from build123d import *

# Parameters (mm, degrees)
F1_DEPTH = 60
F2_SIZE  = 40
F3_R     = 90
F4_DEPTH = 10
F5_W     = 43
F5_H     = 43
F6_DEPTH = 40
F7_R     = 4
F8_DEPTH = 10


with BuildPart() as f1:
    # F0 (on Top) → F1 (new body)
    with BuildSketch(Plane.XY):
        Polygon((-173.205081, -100), (173.205081, -100), (0, 200), align=None)
    extrude(amount=F1_DEPTH)

    # F2
    f2_edges = [f1.edges().sort_by_distance(p)[0] for p in [
        (-173.205081, -100, 30),
        (173.205081, -100, 30),
        (0, 200, 30),
    ]]
    chamfer(f2_edges, length=F2_SIZE)

    # F3 (on face) → F4 (join)
    with BuildSketch(Plane.XY.offset(60)):
        Circle(F3_R)
    extrude(amount=F4_DEPTH)

    # F5 (on face) → F6 (cut)
    with BuildSketch(Plane.XY.offset(60)):
        with Locations((0, 130.358984)):
            Rectangle(F5_W, F5_H)
        Polygon((-120.763738, -94.549038), (-83.524645, -73.049038), (-105.024645, -35.809946), (-142.263738, -57.309946), align=None)
        Polygon((142.263738, -57.309946), (105.024645, -35.809946), (83.524645, -73.049038), (120.763738, -94.549038), align=None)
    extrude(amount=-F6_DEPTH, mode=Mode.SUBTRACT)

    # F7 (on face) → F8 (cut)
    with BuildSketch(Plane.XY.offset(60)):
        with Locations((-29.5, 130.358984)):
            Circle(F7_R)
        with Locations((29.5, 130.358984)):
            Circle(F7_R)
        with Locations((-98.144192, -90.727241)):
            Circle(F7_R)
        with Locations((-127.644192, -39.631743)):
            Circle(F7_R)
        with Locations((127.644192, -39.631743)):
            Circle(F7_R)
        with Locations((98.144192, -90.727241)):
            Circle(F7_R)
    extrude(amount=-F8_DEPTH, mode=Mode.SUBTRACT)


solid = f1.part
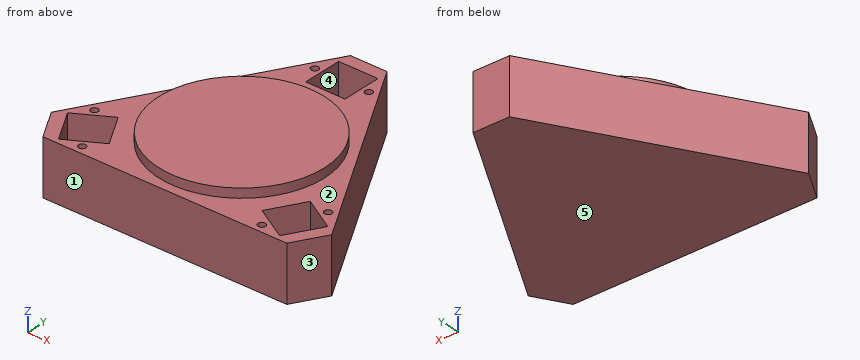
Verification items for the finished model (mm, model axes). Face numbers are marked on the shaded views. A direction names the side the tool comes from. Coordinates: 2 decimals unless noted, no trailing zeros. Loops run counter-clockwise (first coordinate to the right, second up) from the corner with the lowest first, then second, coordinate; pieces in that order, holes last. Notation, with made-up numbers: M 6,26 L 19,26 A12 cw 19,31 Z; hole C -39,46.25 d10. An arc over 180 degrees is marked long. One line per item, written item: value.
1. Section check A-A on z = 29.5. Record the cut outline in (x, y), plus the area to 3 significant figures.
Answers follow:
outline: M -153.21,-65.36 L -133.21,-100 L 133.21,-100 L 153.21,-65.36 L 20,165.36 L -20,165.36 Z; hole M -142.26,-57.31 L -120.76,-94.55 L -83.52,-73.05 L -105.02,-35.81 Z; hole M -21.5,108.86 L 21.5,108.86 L 21.5,151.86 L -21.5,151.86 Z; hole M 83.52,-73.05 L 120.76,-94.55 L 142.26,-57.31 L 105.02,-35.81 Z
area: 44,300 mm^2
2. Gauge pin test, flat ends, axial feed: P1, Ø13, axis at x = -98.14, y = -90.73, coming from the +Z side; P2, Ø2.5, axis at x = -129, y = -39, coming from the +Z side; P3, Ø5, axis at y = 112.5, z = 57, coming from the +X side. Record the tip position at first contact, or that the pin passes through.
Answers follow:
P1: z = 60
P2: z = 50
P3: x = 51.96
3. Mould release check, pull along Y, two halves, no side actions. Record for the marked faces 3, 4 and 5: pulls with the +Y half, pulls with the -Y half, needs draft (parallel to the pull), parting line crosses it, or undercut.
Answers follow:
face 3: pulls with the -Y half
face 4: undercut
face 5: needs draft
4. Section check B-B on x = 0. Record the cut outline in (y, z), plus the area to 3 significant figures.
Answers follow:
outline: M -100,0 L 165.36,0 L 165.36,60 L 151.86,60 L 151.86,20 L 108.86,20 L 108.86,60 L 90,60 L 90,70 L -90,70 L -90,60 L -100,60 Z
area: 16,000 mm^2
5. Section check C-C on y = 37. Record the cut outline in (x, z).
Answers follow:
outline: M -94.11,0 L 94.11,0 L 94.11,60 L 82.04,60 L 82.04,70 L -82.04,70 L -82.04,60 L -94.11,60 Z
6. Set-up check for the marked faces 1 and 2: record each of +Z, -Z, +X, -X, +Y, -Y from which the full face is reachable in a straight line by a thin tool's end or side.
Answers follow:
face 1: +Z, -Z, +X, -X, -Y
face 2: +Z
7. Section check D-D on z = 63.5. Record the cut outline in (x, y).
Answers follow:
outline: C 0,0 d180
8. Material ranges on line 1 along X through (y, z) = (-45, 41); line 2 along Y through (x, z) = (18, 50.5); line 3 along Y through (x, z) = (29.5, 56), recorded low to high. Write a range as from..to.
Answers follow:
line 1: -141.45..-120.94, -99.72..99.72, 120.94..141.45
line 2: -100..108.86, 151.86..165.36
line 3: -100..126.36, 134.36..148.9
